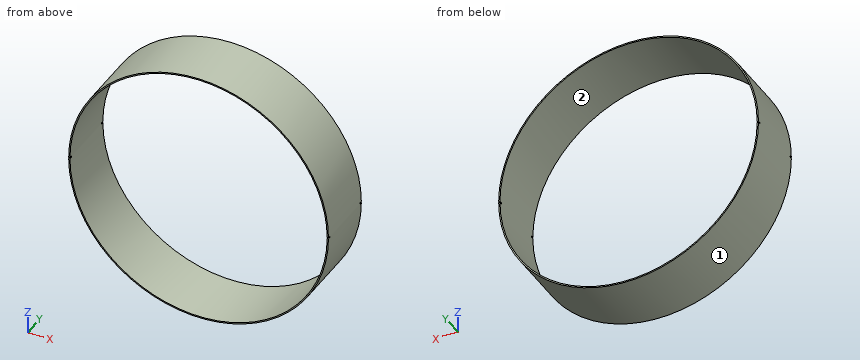
from build123d import *

# Parameters (mm, degrees)
SKETCH_1_R               = 50.3
SKETCH_1_R_2             = 49.8
EXTRUDE_1_DEPTH          = 24
CUT_EXTRUDE_2_DEPTH      = 52
CUT_EXTRUDE_2_DEPTH_BACK = 52


with BuildPart() as part:
    # Sketch 1 → Extrude 1 (new body)
    with BuildSketch(Plane(origin=(0, 0, 0), x_dir=(1, 0, 0), z_dir=(0, 1, 0))):
        with Locations(Location((0, 0, 0), (0, 0, 270))):
            Circle(SKETCH_1_R)
        with Locations(Location((0, 0, 0), (0, 0, 270))):
            Circle(SKETCH_1_R_2, mode=Mode.SUBTRACT)
    extrude(amount=EXTRUDE_1_DEPTH)

    # Sketch 3 → Cut-Extrude 2 (cut, two sides: drawn at the far end of the back side and taken through both)
    with BuildSketch(Plane(origin=(0, 0, 0), x_dir=(0, 0, -1), z_dir=(1, 0, 0)).offset(-CUT_EXTRUDE_2_DEPTH_BACK)):
        Polygon((0, 24), (0.25, 24), (0.25, 23), (-0.25, 23), (-0.25, 24), align=None)
        Polygon((0.25, 1), (0.25, 0), (0, 0), (-0.25, 0), (-0.25, 1), align=None)
    extrude(amount=CUT_EXTRUDE_2_DEPTH + CUT_EXTRUDE_2_DEPTH_BACK, mode=Mode.SUBTRACT)


solid = part.part
Can you work these out from the model? Positions are in its coordinate system, mm. Face numbers are marked on the shaded views. Round coordinates to 2 decimals unless told otherwise and drop trailing zeros. Loops run counter-clockwise (first coordinate to the right, second up) from the corner with the lowest first, then second, coordinate; pieces in that order, holes last. Notation, with made-up numbers: (-3.5, -23.5) - (37.5, -23.5) arc R38 cw to (37.5, 15.5) - close; hole circle Ø7 at (13, 23). An arc over 180 degrees is marked (long way). Answer in a Markdown table with one row per item. Add a question column.
Q1. I want a section at B-B on z = 9.5. List the corners of the cut face in (x, y) for me, and give its area (3 significant figures).
Q2. We'd pull the mould along Z, two halves only. Please class the marked faces 1 and 2: pulls with the +Z half, pulls with the -Z half, needs draft (parallel to the pull), parting line crosses it, or undercut.
Q3. I want a section at C-C on y = 5. List the corners of the cut face in (x, z) for me.
Q4. I need wall thicknesses on L1, parallel to Z at x = 0, y = 12; L2, parallel to X at y = 4, z = -25. Which ranges of each line are inside material? Lowest first, please.
Q5. I want a section at A-A on x = 0. List the corners of the cut face in (y, z) for me.
Q6. For pin 1 Ø4 at (y, z) = (4, 23) entering from -X; pin 2 Ø10 at (y, z) = (15, 7.5) entering from -X; pin 3 Ø6 at (x, y) = (12, 5.5) entering from +Z, each with a flat end and sliding along its axis, tell me the tip position at first contact or that it passes through.
A:
| question | item | result |
|---|---|---|
| 1 | outline | (-49.39, 0) - (-48.89, 0) - (-48.89, 24) - (-49.39, 24) - close; (48.89, 0) - (49.39, 0) - (49.39, 24) - (48.89, 24) - close |
| 1 | area | 24.4 mm^2 |
| 2 | face 1 | parting line crosses it |
| 2 | face 2 | undercut |
| 3 | outline | circle Ø100.6 at (0, 0); hole circle Ø99.6 at (0, 0) |
| 4 | L1 | -50.3 to -49.8, 49.8 to 50.3 |
| 4 | L2 | -43.65 to -43.07, 43.07 to 43.65 |
| 5 | outline | (0, -50.3) - (24, -50.3) - (24, -49.8) - (0, -49.8) - close; (0, 49.8) - (24, 49.8) - (24, 50.3) - (0, 50.3) - close |
| 6 | pin 1 | x = -45.71 |
| 6 | pin 2 | x = -50.24 |
| 6 | pin 3 | z = 49.49 |
